Geometry: final body of the model. Coordinates: model frame, mm. Coordinates: 2 decimals unless noted, no trailing zeros. Order: outer loops, then holes, each group sorted by start corner. A loop starts at its lowest first (then second) coordinate and runs counter-clockwise, first axis right, second up. Notation, with made-up numbers: (80.25, 34) - (117.25, 34) arc R5 ccw to (117.25, 41) - close; hole circle Ø2 at (-32, 9). An arc over 180 degrees is marked (long way). Use one line per item in the form item = value. Start each with the question number.
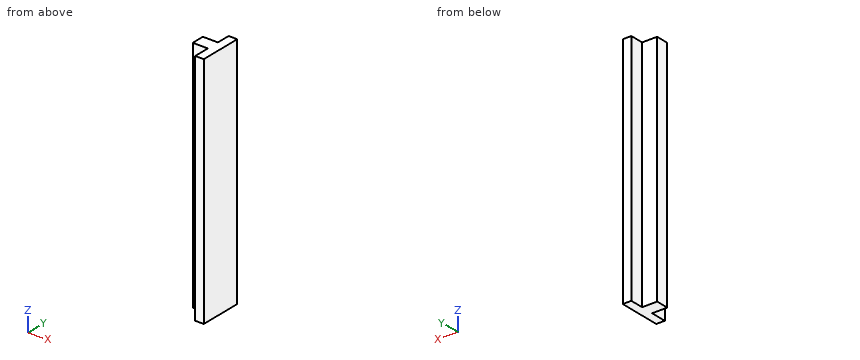
```python
from build123d import *

# Parameters (mm, degrees)
EXTRUDE2_DEPTH = 137.5


with BuildPart() as part:
    # Sketch1 → Extrude2 (new body)
    with BuildSketch(Plane.XY.offset(-35.173777659)):
        Polygon((85.961408719, 43.751957214), (94.761408719, 43.751957214), (94.761408719, 51.676244301), (99.761408719, 51.676244301), (99.761408719, 27.051957214), (94.761408719, 27.051957214), (94.761408719, 36.351957214), (85.961408719, 36.351957214), align=None)
    extrude(amount=-EXTRUDE2_DEPTH)


solid = part.part
```
(1) Contact query for flat-ended pins moving along their axis: pin 1 Ø1.5 at (y, z) = (48, -62.5) entering from -X; pin 2 Ø4.5 at (x, z) = (91.5, -73) entering from +Y; pin 3 Ø3 at (x, z) = (88.5, -158.5) entering from -Y. Output: stop coordinate, or through.
(2) Material intervals for L1, parallel to X at y = 48.75, z = -124.5; L2, parallel to Y at x = 88, z = -76, sorted ascending. Write a range as from..to.
(3) Cut plane C-C on y = 29.25. Return the cut outline in (x, z), plus the area to 4 significant figures.
(4) Cut plane A-A on z = -57. Return the cut outline in (x, y).
(5) Cut plane B-B on x = 91.25. Return the cut outline in (y, z), plus the area to 3 significant figures.
Check sheet entries:
q1.pin_1 = 94.76
q1.pin_2 = 43.75
q1.pin_3 = 36.35
q2.L1 = 94.76..99.76
q2.L2 = 36.35..43.75
q3.outline = (94.76, -172.67) - (99.76, -172.67) - (99.76, -35.17) - (94.76, -35.17) - close
q3.area = 687.5 mm^2
q4.outline = (85.96, 36.35) - (94.76, 36.35) - (94.76, 27.05) - (99.76, 27.05) - (99.76, 51.68) - (94.76, 51.68) - (94.76, 43.75) - (85.96, 43.75) - close
q5.outline = (36.35, -172.67) - (43.75, -172.67) - (43.75, -35.17) - (36.35, -35.17) - close
q5.area = 1,020 mm^2
